Work out the finished part from the listing and answer in its coordinate system (mm). Give positions to 0.01 mm unless a question says otherwise; leave off trailing zeros. Write each loop counter-clockwise with the first axis right and the second up, starting at its lowest first coordinate (ties: lowest second). Pieces come first, ordered by that corner, then holes.
1) Given pin 1 Ø1.5 at (x, y) = (209.5, 72) entering from -Z, flat-ended and moving along its own axis, determine where the tip first touches the part or whether it passes through.
2) Find section B-B (z = 2.55). Determine the outline of the cut face in (x, y), plus the area to 3 significant figures.
3) Find section D-D (y = 70.5). Determine the outline of the cut face in (x, z).
4) Straight lines are drawn through the part: probe 1 along Y at (x, z) = (148.5, 1.5); probe 2 along X at (y, z) = (125, 2.45); probe 3 along Y at (x, z) = (15, 2.65). For each, find the intervals that lie inside material, in ascending order.
5) Find section C-C (y = 54.9). Determine the outline of the cut face in (x, z), plus the area to 3 significant figures.
6) Determine the mould class of faces 1 (the face through (232.04, 63.14, 1.48)), 2 (the face through (117, 63, 0)), 3 (the face through (23.3, 121.72, 1.48)) for opening direction Y: pulls with the +Y half, pulls with the -Y half, needs draft (parallel to the pull), parting line crosses it, or undercut.
7) Find section A-A (x = 108.5). Determine the outline of the cut face in (y, z).
Autodesk Inventor part; units mm, degrees
ref_plane "YZ Plane" through (0, 0, 0) normal (1, 0, 0) x (0, 1, 0)
ref_plane "XZ Plane" through (0, 0, 0) normal (0, 1, 0) x (-1, 0, 0)
ref_plane "XY Plane" through (0, 0, 0) normal (0, 0, 1) x (1, 0, 0)
sketch "Sketch1" plane through (0, 0, 0) normal (0, 0, 1) x (1, 0, 0)
  line L0 (0, 0) -> (237, 0)
  line L1 (10.5075, 133.75) -> (226.4925, 133.75)
  line L2 (10.5075, 133.75) -> (0, 0)
  line L3 (226.4925, 133.75) -> (237, 0)
  circle A0 centre (25.5075, 123.75) radius 3
  line L4 (118.5, 191.0895) -> (118.5, 206.5913) construction
  circle A1 centre (211.4925, 123.75) radius 3
  line L5 (28.5, 54.9) -> (208.5, 54.9) construction
  line L6 (28.5, 51.8) -> (208.5, 51.8)
  line L7 (208.5, 58) -> (28.5, 58)
  arc A2 (28.5, 58) -> (28.5, 51.8) centre (28.5, 54.9) ccw
  arc A3 (208.5, 51.8) -> (208.5, 58) centre (208.5, 54.9) ccw
  point P0 (118.5, 133.75)
  point P1 (118.5, 0)
  point P2 (118.5, 198.8404)
  point P3 (118.5, 54.9)
  dimension "d0" = 237
  dimension "d1" = 215.985
  dimension "d2" = 133.75
  dimension "d3" = 6
  dimension "d4" = 10
  dimension "d5" = 15
  dimension "d8" = 6.2
  dimension "d9" = 81.95
  dimension "d10" = 180
extrude "Extrusion1" add sketch "Sketch1" along normal blind 3
sketch "Sketch2" plane through (0, 0, 3) normal (0, 0, 1) x (1, 0, 0)
  line L0 (0, 0) -> (237, 0)
  line L1 (237, 0) -> (237, -9)
  line L2 (237, -9) -> (0, -9)
  line L3 (0, -9) -> (0, 0)
  dimension "depth" = 9
extrude "Extrusion2" add sketch "Sketch2" against normal blind 3
fillet "Fillet1" radius 10 2 edges at (226.4925, 133.75, 1.5) (10.5075, 133.75, 1.5)
sketch "Sketch3" plane through (0, 0, 3) normal (0, 0, 1) x (1, 0, 0)
  line L0 (0, 0) -> (0, -9)
  line L1 (0, -9) -> (237, -9)
  spline S0 degree 4 poles (208.9384, 106.1179) (205.6345, 87.6966) (186.3734, 52.9377) (139.2784, 16.5104) (82.7331, 6.5959) (51.8588, 6.1179) knots 0 0 0 0 0 0.457223 1 1 1 1 1
  point P0 (199.8798, 81.1179)
  point P1 (180.3986, 56.1179)
  point P2 (147.52, 31.1179)
  point P3 (103.0387, 12.8166)
equation "\"raisedheight\" = 5"
equation "\"geargap\" = 0.2"
properties part number "mountback"
Results:
1. pin 1: stops at z = 0
2. outline: (0, -9) - (237, -9) - (237, 0) - (227.22, 124.53) arc R10 ccw to (217.25, 133.75) - (19.75, 133.75) arc R10 ccw to (9.78, 124.53) - (0, 0) - close; hole circle Ø6 at (25.51, 123.75); hole (28.5, 51.8) - (208.5, 51.8) arc R3.1 ccw to (208.5, 58) - (28.5, 58) arc R3.1 ccw to start; hole circle Ø6 at (211.49, 123.75)
2. area: 31,200 mm2
3. outline: (5.54, 0) - (231.46, 0) - (231.46, 3) - (5.54, 3) - close
4. probe 1: y = -9 to 51.8, 58 to 133.75
4. probe 2: x = 9.83 to 22.78, 28.23 to 208.77, 214.22 to 227.17
4. probe 3: y = -9 to 132.55
5. outline: (4.31, 0) - (25.4, 0) - (25.4, 3) - (4.31, 3) - close; (211.6, 0) - (232.69, 0) - (232.69, 3) - (211.6, 3) - close
5. area: 127 mm2
6. face 1: pulls with the +Y half
6. face 2: needs draft
6. face 3: undercut
7. outline: (-9, 0) - (51.8, 0) - (51.8, 3) - (-9, 3) - close; (58, 0) - (133.75, 0) - (133.75, 3) - (58, 3) - close
